from build123d import *

# Parameters (mm, degrees)
F1_DEPTH = 31.75
F2_R     = 3.175
F3_DEPTH = 41.402
F2_R_2   = 7.9375
F4_DEPTH = 12.7


with BuildPart() as f1:
    # F0 (on Front) → F1 (new body, symmetric)
    with BuildSketch(Plane.XZ):
        with BuildLine():
            Line((-31.75, 0), (-19.05, 0))
            ThreePointArc((-19.05, 0), (0, 19.05), (19.05, 0))
            Line((19.05, 0), (31.75, 0))
            ThreePointArc((31.75, 0), (0, 31.75), (-31.75, 0))
        make_face()
    extrude(amount=F1_DEPTH, both=True)

    # F2 (on Top) → F3 (cut)
    with BuildSketch(Plane.XY):
        Circle(F2_R)
    extrude(amount=F3_DEPTH, mode=Mode.SUBTRACT)

    # F2 (on Top) → F4 (join)
    with BuildSketch(Plane.XY):
        with BuildLine():
            ThreePointArc((82.514942, -19.076727), (101.564942, -0.026727), (82.514942, 19.023273))
            Line((82.514942, 19.023273), (19.05, 19.023273))
            Line((19.05, 19.023273), (19.05, -19.076727))
            Line((19.05, -19.076727), (82.514942, -19.076727))
        make_face()
        with Locations((82.514942, -0.026727)):
            Circle(F2_R_2, mode=Mode.SUBTRACT)
        with BuildLine():
            Line((-19.05, 19.443342), (-81.509791, 19.443342))
            ThreePointArc((-81.509791, 19.443342), (-100.559791, 0.393342), (-81.509791, -18.656658))
            Line((-81.509791, -18.656658), (-19.05, -18.656658))
            Line((-19.05, -18.656658), (-19.05, 19.443342))
        make_face()
        with Locations((-81.509791, 0.393342)):
            Circle(F2_R_2, mode=Mode.SUBTRACT)
    extrude(amount=F4_DEPTH)


solid = f1.part
Design review of the part built by this model. Coordinates are the model's own, in mm. A direction names the side the tool comes from. Give positions to 0.01 mm unless a question says otherwise; leave off trailing zeros. Order: outer loops, then holes, each group sorted by start corner. A loop starts at its lowest first (then second) coordinate and runs counter-clockwise, first axis right, second up. Notation, with made-up numbers: (29, -5.5) - (81, -5.5) arc R17 cw to (81, 26.5) - close; hole circle Ø7 at (-15.5, 84). An arc over 180 degrees is marked (long way). Write item = value, one per line. Start each with the question number.
Q1. To check wall thickness, follow L1, parallel to Y at x = 0, z = 22.5 (3 decimals); L2, parallel to Z at x = -32, y = -10; L3, parallel to X at y = 21, z = 13. State the ranges of each line that lie inside material, in increasing order. Write a range as from..to.
Q2. Mouldability with a two-part tool opening along Y and no side actions: class faces 3 (the face through (90.086, 2.357, 6.261)), 4 (the face through (-56, -18.657, 6)), 5 (the face through (-0.69, -3.1, 25.18)), 6 (the face through (-65, 1, 12.7)) as released by +Y, released by -Y, zero draft, split by the parting line, or undercut.
Q3. Clearance check with flat-ended pins moving along their axes: pin 1 Ø3 at (y, z) = (-20.5, 23) entering from +X; pin 2 Ø14 at (x, z) = (-59, 8.5) entering from -Y; pin 3 Ø4 at (x, z) = (-54.5, 3.5) entering from +Y; pin 4 Ø6 at (x, z) = (22.5, 27) entering from -Y. State where each tip first meets the part, or that it passes through.
Q4. We need section D-D on y = -26.5. State the section outline as (x, z) points, plus the area to 3 significant figures.
Q5. We need section C-C on z = 15. State the section outline as (x, y) points, plus the area to 3 significant figures.
Q6. We need section B-B on z = 6.5. State how many separate pieces and enclosed holes the cut face has, plus the area to 3 significant figures.
Q7. Tool access review of faces 1 (the face through (65, 0, 12.7)), 2 (the face through (101.56, -0.45, 6.26)): name each direction out of +Z, -Z, +X, -X, +Y, -Y from which nothing blocks a thin tool from reaching the whole face with its end or side.
Q8. We need section A-A on x = 79. State the section outline as (y, z) points.
Working result:
q1.L1 = -31.75..-3.175, 3.175..31.75
q1.L2 = 0..12.7
q1.L3 = -28.97..-13.92, 13.92..28.97
q2.face_3 = undercut
q2.face_4 = released by -Y
q2.face_5 = undercut
q2.face_6 = zero draft
q3.pin_1 = 23.36
q3.pin_2 = -18.66
q3.pin_3 = 19.44
q3.pin_4 = through
q4.outline = (-31.75, 0) - (-19.05, 0) arc R19.05 cw to (19.05, 0) - (31.75, 0) arc R31.75 ccw to start
q4.area = 1,010 mm²
q5.outline = (-27.98, -31.75) - (-11.74, -31.75) - (-11.74, 31.75) - (-27.98, 31.75) - close; (11.74, -31.75) - (27.98, -31.75) - (27.98, 31.75) - (11.74, 31.75) - close
q5.area = 2,060 mm²
q6.separate_pieces = 2
q6.enclosed_holes = 2
q6.area = 6,300 mm²
q7.face_1 = +Z, +X, +Y, -Y
q7.face_2 = +Z, -Z, +X
q8.outline = (-19.08, 0) - (-7.14, 0) - (-7.14, 12.7) - (-19.08, 12.7) - close; (7.09, 0) - (19.02, 0) - (19.02, 12.7) - (7.09, 12.7) - close
